from build123d import *

# Parameters (mm, degrees)
SKETCH1_R           = 101.6
BOSS_EXTRUDE1_DEPTH = 22.352
SKETCH2_R           = 34.925
BOSS_EXTRUDE2_DEPTH = 12.7
SKETCH3_R           = 22.352
BOSS_EXTRUDE3_DEPTH = 41.148
SKETCH4_R           = 20.6375
CUT_EXTRUDE1_DEPTH  = 158.090324336


with BuildPart() as part:
    # Sketch1 → Boss-Extrude1 (new body)
    with BuildSketch(Plane(origin=(0, 0, 0), x_dir=(1, 0, 0), z_dir=(0, 1, 0))):
        with Locations(Location((0, 0, 0), (0, 0, 270))):
            Circle(SKETCH1_R)
    extrude(amount=BOSS_EXTRUDE1_DEPTH)



with BuildPart() as body_2:
    # Sketch2 → Boss-Extrude2 (new body)
    with BuildSketch(Plane.XZ.offset(-63.5)):
        with Locations(Location((0, 0, 0), (0, 0, 270))):
            Circle(SKETCH2_R)
    extrude(amount=BOSS_EXTRUDE2_DEPTH)


with BuildPart() as part_1:
    add(part.part)

    add(body_2.part)  # Boss-Extrude3 merges body 2
    # Sketch3 → Boss-Extrude3 (add)
    with BuildSketch(Plane(origin=(0, 63.5, 0), x_dir=(1, 0, 0), z_dir=(0, 1, 0))):
        with Locations(Location((0, 0, 0), (0, 0, 270))):
            Circle(SKETCH3_R)
    extrude(amount=-BOSS_EXTRUDE3_DEPTH)

    # Sketch4 → Cut-Extrude1 (cut, through all)
    with BuildSketch(Plane(origin=(0, 63.5, 0), x_dir=(1, 0, 0), z_dir=(0, 1, 0))):
        with Locations(Location((0, 0, 0), (0, 0, 270))):
            Circle(SKETCH4_R)
    extrude(amount=-CUT_EXTRUDE1_DEPTH, mode=Mode.SUBTRACT)


solid = part_1.part
Work out the finished part from the listing and answer in its coordinate system (mm). A direction names the side the tool comes from. Give positions to 0.01 mm unless a question says otherwise; leave off trailing zeros. Loops run counter-clockwise (first coordinate to the right, second up) from the corner with the lowest first, then second, coordinate; pieces in that order, holes last. Notation, with made-up numbers: (-26, 58) - (18, 58) arc R22 ccw to (18, 73) - close; hole circle Ø9 at (52, -35.5). An arc over 180 degrees is marked (long way). Answer in a Markdown table with one row per item. Add a question column.
Q1. Consider line 1 along Y through (x, z) = (-26, 19.5); line 2 along X through (y, z) = (18, 0); line 3 along X through (y, z) = (46.5, 0). Determine where each line is inside the solid, lowest interval first.
Q2. Determine the mould class of faces 1 (the cylindrical face through (20.46, 32.19, -2.69)), 2 (the flat face through (-23, 50.8, 0)), 3 (the flat face through (1, 0, 21)) for opening direction Y: released by +Y, released by -Y, zero draft, split by the parting line, or undercut.
Q3. The part is cut by section B-B (z = 0). Determine the outline of the cut face in (x, y) (1 decimal), and give its area (3 significant figures).
Q4. A tool of negligible diameter and unlimited length cuts with its end or side. For faces 4 (the cylindrical face through (-34.094, 57.239, 7.571)), 5 (the cylindrical face through (-21.82, 36.78, -4.85)), 6 (the cylindrical face through (-61.82, 11.02, -80.63)), from which of +Z, -Z, +X, -X, +Y, -Y can it reach the whole face along a straight path? Write none if from no direction.
Q5. The part is cut by section D-D (x = -63). Determine the outline of the cut face in (y, z), and give its area (3 significant figures).
Q6. Each of these flat-tipped pins is pushed along its axis until it touches: P1, Ø12, axis at x = 37.5, y = 25, coming from the -Z side; P2, Ø2, axis at x = 41.5, z = -41, coming from the +Y side; P3, Ø12, axis at x = 20.5, y = 24.5, coming from the -Z side. Where does it stop, or does it pass through?
Q7. The part is cut by section A-A (x = 0). Determine the outline of the cut face in (y, z) (1 decimal), and give its area (3 significant figures).
Q8. The part is cut by section C-C (y = 5). Determine the outline of the cut face in (x, z) (1 decimal).
Solution:
| question | item | result |
|---|---|---|
| 1 | line 1 | y = 0 to 22.35, 50.8 to 63.5 |
| 1 | line 2 | x = -101.6 to -20.64, 20.64 to 101.6 |
| 1 | line 3 | x = -22.35 to -20.64, 20.64 to 22.35 |
| 2 | face 1 | zero draft |
| 2 | face 2 | undercut |
| 2 | face 3 | released by -Y |
| 3 | outline | (-101.6, 0) - (-20.6, 0) - (-20.6, 63.5) - (-34.9, 63.5) - (-34.9, 50.8) - (-22.4, 50.8) - (-22.4, 22.4) - (-101.6, 22.4) - close; (20.6, 0) - (101.6, 0) - (101.6, 22.4) - (22.4, 22.4) - (22.4, 50.8) - (34.9, 50.8) - (34.9, 63.5) - (20.6, 63.5) - close |
| 3 | area | 4,080 mm² |
| 4 | face 4 | +Y |
| 4 | face 5 | none |
| 4 | face 6 | +Y, -Y |
| 5 | outline | (0, -79.71) - (22.35, -79.71) - (22.35, 79.71) - (0, 79.71) - close |
| 5 | area | 3,560 mm² |
| 6 | P1 | stops at z = -96.39 |
| 6 | P2 | stops at y = 22.35 |
| 6 | P3 | stops at z = -100.5 |
| 7 | outline | (0, -101.6) - (22.4, -101.6) - (22.4, -22.4) - (50.8, -22.4) - (50.8, -34.9) - (63.5, -34.9) - (63.5, -20.6) - (0, -20.6) - close; (0, 20.6) - (63.5, 20.6) - (63.5, 34.9) - (50.8, 34.9) - (50.8, 22.4) - (22.4, 22.4) - (22.4, 101.6) - (0, 101.6) - close |
| 7 | area | 4,080 mm² |
| 8 | outline | circle Ø203.2 at (0, 0); hole circle Ø41.3 at (0, 0) |
